from build123d import *

# Parameters (mm, degrees)
F0_W     = 1905
F0_H     = 584.2
F0_W_2   = 279.4
F0_H_2   = 152.4
F0_W_3   = 368.3
F0_H_3   = 101.6
F0_W_4   = 84.16
F0_H_4   = 55.16
F0_W_5   = 127
F0_H_5   = 127
F0_W_6   = 161.8
F0_H_6   = 85.6
F0_W_7   = 355.6
F0_H_7   = 88.9
F0_H_8   = 215.9
F0_W_8   = 266.7
F0_H_9   = 139.7
F0_W_9   = 149.1
F0_H_10  = 72.9
F0_W_10  = 150.6218942523
F0_W_11  = 95.475
F0_H_11  = 6.35
F0_H_12  = 4.8625
F1_DEPTH = 6.35
F2_D     = 4.1656
F3_D     = 7.0104
F4_D     = 54
F5_D     = 86


# Not quite as in the source:
# - a feature names something its author has since deleted; it is built from what else it names


with BuildPart() as f1:
    # F0 (on Top) → F1 (new body)
    with BuildSketch(Plane.XY):
        with Locations((499.8503303409, 41.4113755345)):
            Rectangle(F0_W, F0_H)
        with Locations((455.4003303409, 16.0113749921)):
            Rectangle(F0_W_2, F0_H_2, mode=Mode.SUBTRACT)
        with Locations((1179.3003303409, -9.3886244655)):
            Rectangle(F0_W_3, F0_H_3, mode=Mode.SUBTRACT)
        with Locations((185.112135537, 77.3313755345)):
            Rectangle(F0_W_4, F0_H_4, mode=Mode.SUBTRACT)
        with Locations((-33.5496696591, 244.6113755345)):
            Rectangle(F0_W_5, F0_H_5, mode=Mode.SUBTRACT)
        Polygon((315.7003303409, 314.4613755345), (315.7003303409, 320.8113755345), (411.1753303409, 320.8113755345), (411.1753303409, 314.4613755345), (414.1253303409, 314.4613755345), (414.1253303409, 246.1988755345), (411.1753303409, 246.1988755345), (411.1753303409, 241.3363755345), (315.7003303409, 241.3363755345), (315.7003303409, 246.1988755345), align=None, mode=Mode.SUBTRACT)
        Polygon((639.5503303409, 54.1113755345), (639.5503303409, 168.4113755345), (931.6503303409, 168.4113755345), (931.6503303409, -60.1886244655), (785.6003303409, -60.1886244655), (639.5503303409, -60.1886244655), align=None, mode=Mode.SUBTRACT)
        with Locations((1076.0503303409, 122.3113755345)):
            Rectangle(F0_W_6, F0_H_6, mode=Mode.SUBTRACT)
        with Locations((1282.5503303409, 122.3113742352)):
            Rectangle(F0_W_6, F0_H_6, mode=Mode.SUBTRACT)
        Polygon((496.6753303409, 314.4613755345), (496.6753303409, 320.8113755345), (592.1503303409, 320.8113755345), (592.1503303409, 314.4613755345), (595.1003303409, 314.4613755345), (595.1003303409, 246.1988755345), (592.1503303409, 246.1988755345), (592.1503303409, 241.3363755345), (496.6753303409, 241.3363755345), (496.6753303409, 246.1988755345), align=None, mode=Mode.SUBTRACT)
        with Locations((1179.3003303409, -9.3886244655)):
            Rectangle(F0_W_3, F0_H_3)
        with Locations((1179.3003303409, -9.3886244655)):
            Rectangle(F0_W_7, F0_H_7, mode=Mode.SUBTRACT)
        Polygon((931.6503303409, 168.4113755345), (639.5503303409, 168.4113755345), (639.5503303409, 54.1113755345), (639.5503303409, -60.1886244655), (785.6003303409, -60.1886244655), (931.6503303409, -60.1886244655), align=None)
        with Locations((785.6003303409, 54.1113755345)):
            Rectangle(F0_W_2, F0_H_8, mode=Mode.SUBTRACT)
        with Locations((455.4003303409, 16.0113749921)):
            Rectangle(F0_W_2, F0_H_2)
        with Locations((455.4003303409, 16.0113749921)):
            Rectangle(F0_W_8, F0_H_9, mode=Mode.SUBTRACT)
        with Locations((1076.0503303409, 122.3113755345)):
            Rectangle(F0_W_6, F0_H_6)
        with Locations((1076.0503303409, 122.3113755345)):
            Rectangle(F0_W_9, F0_H_10, mode=Mode.SUBTRACT)
        with Locations((1282.5503303409, 122.3113742352)):
            Rectangle(F0_W_6, F0_H_6)
        with Locations((1281.7893832147, 122.3113742352)):
            Rectangle(F0_W_10, F0_H_10, mode=Mode.SUBTRACT)
        with Locations((363.4378303409, 317.6363755345)):
            Rectangle(F0_W_11, F0_H_11)
        with Locations((363.4378303409, 243.7676255345)):
            Rectangle(F0_W_11, F0_H_12)
        with Locations((544.4128303409, 317.6363755345)):
            Rectangle(F0_W_11, F0_H_11)
        with Locations((544.4128303409, 243.7676255345)):
            Rectangle(F0_W_11, F0_H_12)
    extrude(amount=F1_DEPTH)

    # F2 (through all)
    with Locations(Plane(origin=(0, 0, 0), x_dir=(1, 0, 0), z_dir=(0, 0, -1))):
        with Locations((995.1503303409, -41.4113755345), (995.1503303409, -7.6293755345), (995.1503303409, 26.1526244655), (995.1503303409, 60.1886244655), (1047.7283303409, 60.1886244655), (1100.3063303409, 60.1886244655), (1152.8843303409, 60.1886244655), (1205.4623303409, 60.1886244655), (1258.0403303409, 60.1886244655), (1310.6183303409, 60.1886244655), (1363.4503303409, 60.1886244655), (1363.4503303409, 26.4066244655), (1363.4503303409, -7.6293755345), (1363.4503303409, -41.4113755345), (1310.6183303409, -41.4113755345), (1258.0403303409, -41.4113755345), (1205.4623303409, -41.4113755345), (1152.8843303409, -41.4113755345), (1100.3063303409, -41.4113755345), (1047.7283303409, -41.4113755345), (639.5503303409, -168.4113755345), (785.6003303409, -168.4113755345), (931.6503303409, -168.4113755345), (931.6503303409, -54.1113755345), (931.6503303409, 60.1886244655), (785.6003303409, 60.1886244655), (639.5503303409, 60.1886244655), (639.5503303409, -54.1113755345), (315.7003303409, -92.2113749921), (455.4003303409, -92.2113749921), (595.1003303409, -92.2113749921), (595.1003303409, 60.1886250079), (455.4003303409, 60.1886250079), (315.7003303409, 60.1886250079), (315.7003303409, -320.8113755345), (411.1753303409, -320.8113755345), (411.1753303409, -241.3363755345), (315.7003303409, -241.3363755345), (496.6753303409, -320.8113755345), (496.6753303409, -241.3363755345), (592.1503303409, -241.3363755345), (592.1503303409, -320.8113755345), (135.614335537, -107.9269755345), (234.614335537, -107.9269755345), (234.614335537, -46.7199755345), (135.614335537, -46.7199755345), (-109.7496696591, -320.8113755345), (-109.7496696591, -168.4113755345), (42.6503303409, -168.4113755345), (42.6503303409, -320.8113755345)):
            Hole(F2_D / 2)

    # F3 (through all)
    with Locations(Plane(origin=(0, 0, 0), x_dir=(1, 0, 0), z_dir=(0, 0, -1))):
        with Locations((995.1503303409, -165.1113755345), (995.1503303409, -79.5113755345), (1156.9503303409, -79.5113755345), (1156.9503303409, -165.1113755345), (1201.6503303409, -165.1113742352), (1201.6503303409, -79.5113742352), (1363.4503303409, -79.5113742352), (1363.4503303409, -165.1113742352)):
            Hole(F3_D / 2)

    # F4 (through all)
    with Locations(Plane(origin=(0, 0, 0), x_dir=(1, 0, 0), z_dir=(0, 0, -1))):
        with Locations((233.1503303409, -181.1113755345), (233.1503303409, -282.7113755345), (131.5503303409, -181.1113755345), (131.5503303409, -282.7113755345)):
            Hole(F4_D / 2)

    # F5 (through all)
    with Locations(Plane(origin=(0, 0, 0), x_dir=(1, 0, 0), z_dir=(0, 0, -1))):
        with Locations((363.4378303409, -165.1363755345), (544.4128303409, -165.1363755345)):
            Hole(F5_D / 2)


solid = f1.part
CAD build for the part. Positions are in the model's coordinates, mm. Give positions to 0.01 mm unless a question says otherwise; leave off trailing zeros. Loops run counter-clockwise (first coordinate to the right, second up) from the corner with the lowest first, then second, coordinate; pieces in that order, holes last. Notation, with made-up numbers: M 33,-11 L 51,-11 A19 cw 51,10 Z; hole C 82,21.5 d2. An arc over 180 degrees is marked long. Answer in a Markdown table with one row per item. Add a question column.
Item 1: Band-saw the part on C-C on z = 1. Give the number of separate pieces and of enclosed holes in the cut face, then the cut area to 3 significant figures.
Item 2: Probe probe 1 along X at (y, z) = (-3.5, 1.5); probe 2 along Y at (x, z) = (1349.5, 1.25); probe 3 along X at (y, z) = (89.5, 3.5). List the from-to ranges inside material, lowest first.
Item 3: Band-saw the part on A-A on x = 1329.5. Give the cut face in (y, z), then the cut area to 3 significant figures.
Item 4: Mould opens along Y. For faces 1 (the face through (151.45, 162.863, 3.219)), 2 (the face through (208.21, 293.05, 3.22)), 3 (the face through (487, 110, 6.35)) say: +Y half, -Y half, draft (parallel to the pull), parting line (faces both ways), or undercut.
Item 5: Band-saw the part on B-B on x = 843.5. Give the cut face in (y, z), then the cut area to 3 significant figures.
Reply:
| question | item | result |
|---|---|---|
| 1 | separate pieces | 1 |
| 1 | enclosed holes | 73 |
| 1 | area | 906,000 mm^2 |
| 2 | probe 1 | x = -452.65 to 322.05, 588.75 to 645.9, 925.3 to 1001.5, 1357.1 to 1452.35 |
| 2 | probe 2 | y = -250.69 to -53.84, 35.06 to 85.86, 158.76 to 333.51 |
| 2 | probe 3 | x = -452.65 to 143.03, 227.19 to 645.9, 925.3 to 1001.5, 1150.6 to 1206.48, 1357.1 to 1452.35 |
| 3 | outline | M -250.69,0 L -53.84,0 L -53.84,6.35 L -250.69,6.35 Z; M 35.06,0 L 85.86,0 L 85.86,6.35 L 35.06,6.35 Z; M 158.76,0 L 333.51,0 L 333.51,6.35 L 158.76,6.35 Z |
| 3 | area | 2,680 mm^2 |
| 4 | face 1 | undercut |
| 4 | face 2 | undercut |
| 4 | face 3 | draft |
| 5 | outline | M -250.69,0 L -53.84,0 L -53.84,6.35 L -250.69,6.35 Z; M 162.06,0 L 333.51,0 L 333.51,6.35 L 162.06,6.35 Z |
| 5 | area | 2,340 mm^2 |
